Drawing for the job (mm, zero at the part's lowest x, y, z). A direction names the side the tool comes from. Coordinates: 2 decimals unless noted, no trailing zeros. Write each loop counter-clockwise with the first axis right and the second up, starting at its lowest first coordinate (ties: lowest second). Pieces come first, ordered by that corner, then holes. Notation, with made-up numbers: M 84.25,49 L 106.25,49 A13 cw 106.25,61 Z; hole C -38.5,25 d11. An arc over 180 degrees is marked long. Use CSV: the item, a comma, the result in double quotes. Start each with the question number.
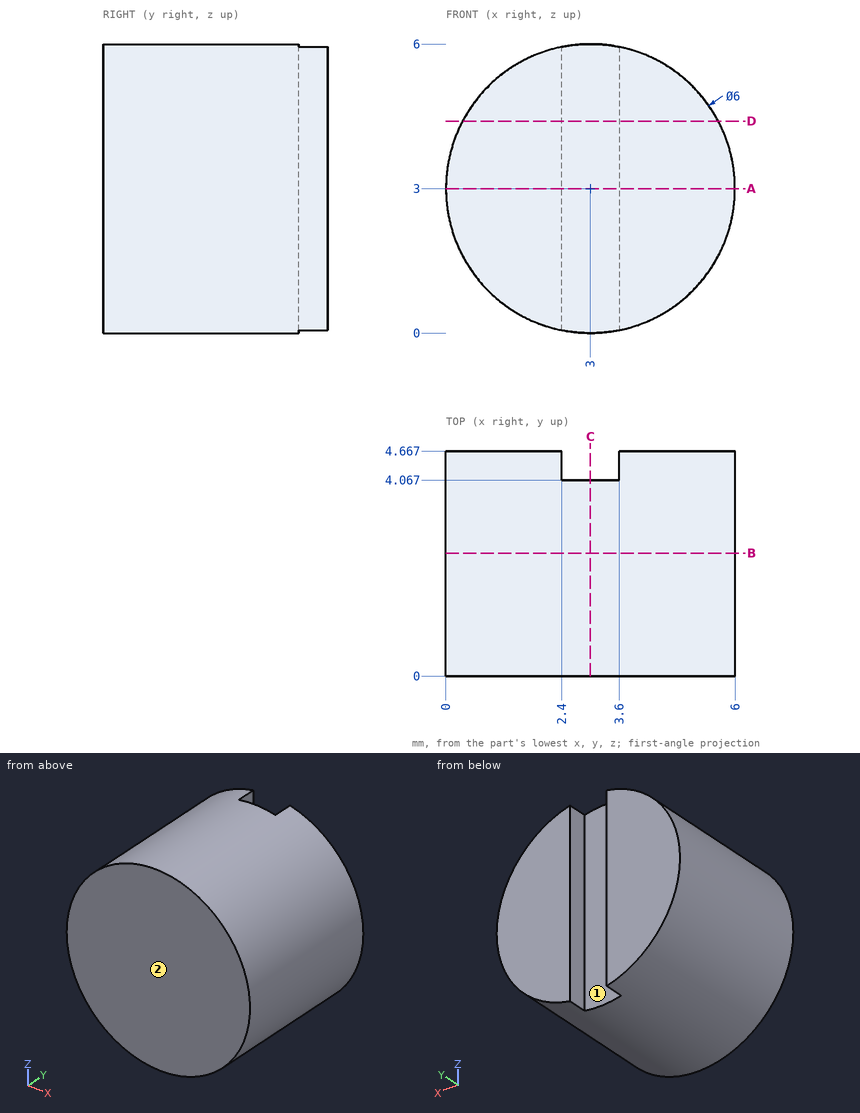
1) Wall check: L1, parallel to X at y = 2.55, z = 3.1; L2, parallel to X at y = 4.3, z = 0.9; L3, parallel to Z at x = 5.5, y = 0.65. Give the ranges that are in metal, low to high. Write a range as [from, to].
2) Band-saw the part on D-D on z = 4.4. List the corners of the cut face in (x, y).
3) Band-saw the part on A-A on z = 3. List the corners of the cut face in (x, y), then the cut area to 3 significant figures.
4) Band-saw the part on B-B on y = 2.55. List the corners of the cut face in (x, z), then the cut area to 3 significant figures.
5) Tool access for the marked faces 1 and 2: list every direction of +Z, -Z, +X, -X, +Y, -Y with a clear straight run to the whole face (end or side of a thin tool).
6) Drop flat-ended pins along their axis: P1, Ø2, axis at y = 3.5, z = 5, coming from the -X side; P2, Ø0.5, axis at y = 4.5, z = 4, coming from the +X side (1 decimal); P3, Ø1.5, axis at x = 2, y = 4, coming from the -Z side. Give the stop position or say it passes through.
7) Band-saw the part on C-C on x = 3. List the corners of the cut face in (y, z).
Findings below:
1,L1,"x = [0, 6]"
1,L2,"x = [0.86, 2.4], [3.6, 5.14]"
1,L3,"z = [1.34, 4.66]"
2,outline,"M 0.35,0 L 5.65,0 L 5.65,4.67 L 3.6,4.67 L 3.6,4.07 L 2.4,4.07 L 2.4,4.67 L 0.35,4.67 Z"
3,outline,"M 0,0 L 6,0 L 6,4.67 L 3.6,4.67 L 3.6,4.07 L 2.4,4.07 L 2.4,4.67 L 0,4.67 Z"
3,area,"27.3 mm2"
4,outline,"C 3,3 d6"
4,area,"28.3 mm2"
5,face 1,"+Z, -Z, +Y"
5,face 2,"+Z, -Z, +X, -X, -Y"
6,P1,"stops at x = 0.17"
6,P2,"stops at x = 5.9"
6,P3,"stops at z = 0.01"
7,outline,"M 0,0 L 4.07,0 L 4.07,6 L 0,6 Z"
